from build123d import *

# Parameters (mm, degrees)
CROQUIS1_W              = 62.313372472
CROQUIS1_H              = 41.924750101
CROQUIS1_W_2            = 60.313372472
CROQUIS1_H_2            = 39.924750101
SALIENTE_EXTRUIR1_DEPTH = 3
CROQUIS3_W              = 1.357711699
CROQUIS3_H              = 39.924750101
CROQUIS3_H_2            = 1
SALIENTE_EXTRUIR2_DEPTH = 18
CROQUIS4_R              = 2.5
CORTAR_EXTRUIR1_DEPTH   = 60.378567465
CROQUIS5_W              = 19.180578122
CROQUIS5_H              = 1.001020226
SALIENTE_EXTRUIR3_DEPTH = 40
CROQUIS6_W              = 27.585602981
CROQUIS6_H              = 16.425068323
CORTAR_EXTRUIR2_DEPTH   = 5
CROQUIS7_W              = 41.924750101
CROQUIS7_H              = 21
CROQUIS7_W_2            = 27.585602981
CROQUIS7_H_2            = 16.425068323
SALIENTE_EXTRUIR4_DEPTH = 25


with BuildPart() as part:
    # Croquis1 → Saliente-Extruir1 (new body)
    with BuildSketch(Plane(origin=(0, 0, 0), x_dir=(1, 0, 0), z_dir=(0, 1, 0))):
        with Locations((31.156686236, 16.749783587)):
            Rectangle(CROQUIS1_W, CROQUIS1_H)
        with Locations((31.156686236, 16.749783587)):
            Rectangle(CROQUIS1_W_2, CROQUIS1_H_2, mode=Mode.SUBTRACT)
    extrude(amount=SALIENTE_EXTRUIR1_DEPTH)

    # Croquis3 → Saliente-Extruir2 (add)
    with BuildSketch(Plane(origin=(0, 3, 0), x_dir=(1, 0, 0), z_dir=(0, 1, 0))):
        with Locations((41.453938501, 16.749783587)):
            Rectangle(CROQUIS3_W, CROQUIS3_H)
        Polygon((42.13279435, -3.212591464), (42.13279435, -4.212591464), (62.313372472, -4.212591464), (62.313372472, 37.712158637), (42.13279435, 37.712158637), (42.13279435, 36.712158637), (61.313372472, 36.712158637), (61.313372472, -3.212591464), align=None)
        with Locations((41.453938501, -3.712591464)):
            Rectangle(CROQUIS3_W, CROQUIS3_H_2)
        with Locations((41.453938501, 37.212158637)):
            Rectangle(CROQUIS3_W, CROQUIS3_H_2)
    extrude(amount=SALIENTE_EXTRUIR2_DEPTH)

    # Croquis4 → Cortar-Extruir1 (cut, through all)
    with BuildSketch(Plane.ZY.offset(-40.775082651)):
        with Locations((-17.242511343, 11.542387771)):
            Circle(CROQUIS4_R)
    extrude(amount=-CORTAR_EXTRUIR1_DEPTH, mode=Mode.SUBTRACT)

    # Croquis5 → Saliente-Extruir3 (add)
    with BuildSketch(Plane.XY.offset(-36.712158637)):
        with Locations((51.723083411, 20.499489887)):
            Rectangle(CROQUIS5_W, CROQUIS5_H)
    extrude(amount=SALIENTE_EXTRUIR3_DEPTH)

    # Croquis6 → Cortar-Extruir2 (cut)
    with BuildSketch(Plane(origin=(62.313372472, 0, 0), x_dir=(0, 0, -1), z_dir=(1, 0, 0))):
        with Locations((17.064754598, 10.282718264)):
            Rectangle(CROQUIS6_W, CROQUIS6_H)
    extrude(amount=-CORTAR_EXTRUIR2_DEPTH, mode=Mode.SUBTRACT)

    # Croquis7 → Saliente-Extruir4 (add)
    with BuildSketch(Plane(origin=(62.313372472, 0, 0), x_dir=(0, 0, -1), z_dir=(1, 0, 0))):
        with Locations((16.749783587, 10.5)):
            Rectangle(CROQUIS7_W, CROQUIS7_H)
        with Locations((17.064754598, 10.282718264)):
            Rectangle(CROQUIS7_W_2, CROQUIS7_H_2, mode=Mode.SUBTRACT)
    extrude(amount=SALIENTE_EXTRUIR4_DEPTH)


solid = part.part
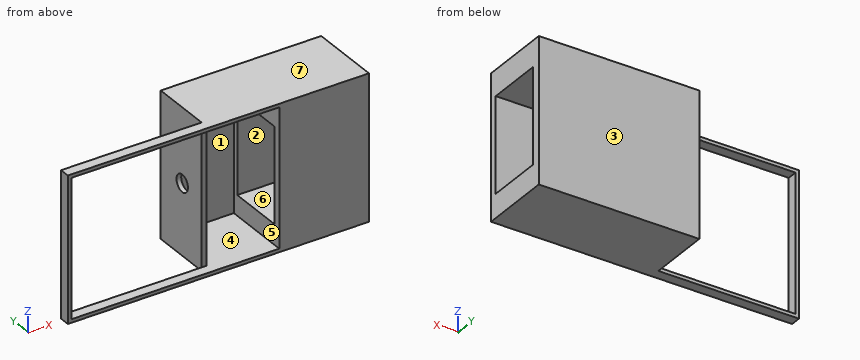
Input: part model. Units: mm. Frame: model coordinates. Face numbers are marked on the shaded views. A direction names the side the tool comes from. Round coordinates to 2 decimals unless told otherwise and drop trailing zeros. Loops run counter-clockwise (first coordinate to the right, second up) from the corner with the lowest first, then second, coordinate; pieces in that order, holes last. Notation, with made-up numbers: M 28,56 L 67,56 A14 cw 67,71 Z; hole C 53,86 d1. An arc over 180 degrees is marked long. Answer as CSV lines item,"result". Start each with the question number.
(1) First-contact query: pin 1 (8 mm diameter, centred on x = 53.5, z = -20.5, fed in from -Y); pin 2 (2 mm diameter, centred on y = 16, z = -26, fed in from +X); pin 3 (2 mm diameter, centred on y = 14, z = -6, fed in from -X). Flat tips, straight axial feed; report the tip coordinate or a pass-through.
(2) Reachability of the marked faces 5, 6 and 7 from +Z, -Z, +X, -X, +Y, -Y: full face, straight path, thin tool, end or side. Return the list, or none.
(3) Section C-C, the plane x = 71. Output: boundary loops of the cut face in (y, z), plus the area to 3 significant figures.
(4) Draft query along Y for the marked faces 1, 2, 3 and 4. Return one class per face: released by +Y, released by -Y, zero draft, split by the parting line, or undercut.
(5) Section B-B, the plane z = -8. Output: boundary loops of the cut face in (x, y), plus the area to 3 significant figures.
(6) Section D-D, the plane y = 4. Output: boundary loops of the cut face in (x, z), plus the area to 3 significant figures.
(7) Section A-A, the plane x = 36.5. Output: boundary loops of the cut face in (y, z).
(8) Line query: line 1 (Z direction, x = 76, y = 4.5); line 2 (X direction, y = 9.75, z = -31); line 3 (Y direction, x = 70, z = -7). Output: solid intervals per line, ascending. Write a range as [from, to].
Values found:
1,pin 1,"stops at y = 20"
1,pin 2,"stops at x = 42.13"
1,pin 3,"stops at x = 40.78"
2,face 5,"-Y"
2,face 6,"+X"
2,face 7,"+Z, +X, -X, +Y, -Y"
3,outline,"M 0,-37.71 L 21,-37.71 L 21,4.21 L 0,4.21 Z; hole M 2.07,-30.86 L 18.5,-30.86 L 18.5,-3.27 L 2.07,-3.27 Z"
3,area,"427 mm²"
4,face 1,"released by -Y"
4,face 2,"undercut"
4,face 3,"released by +Y"
4,face 4,"zero draft"
5,outline,"M 0,0 L 1,0 L 1,3 L 0,3 Z; M 40.78,3 L 42.13,3 L 42.13,20 L 61.31,20 L 61.31,18.5 L 87.31,18.5 L 87.31,21 L 40.78,21 Z; M 61.31,0 L 87.31,0 L 87.31,2.07 L 61.31,2.07 Z"
5,area,"166 mm²"
6,outline,"M 40.78,-37.71 L 87.31,-37.71 L 87.31,-30.86 L 61.31,-30.86 L 61.31,-36.71 L 42.13,-36.71 L 42.13,3.21 L 61.31,3.21 L 61.31,-3.27 L 87.31,-3.27 L 87.31,4.21 L 40.78,4.21 Z"
6,area,"468 mm²"
7,outline,"M 0,-37.71 L 3,-37.71 L 3,-36.71 L 0,-36.71 Z; M 0,3.21 L 3,3.21 L 3,4.21 L 0,4.21 Z"
8,line 1,"z = [-37.71, -30.86], [-3.27, 4.21]"
8,line 2,"x = [40.78, 42.13], [61.31, 87.31]"
8,line 3,"y = [0, 2.07], [18.5, 21]"
